Geometry check sheet. Reference: the model listing, model coordinates, mm. Coordinates: 2 decimals unless noted, no trailing zeros. Order: outer loops, then holes, each group sorted by start corner. A loop starts at its lowest first (then second) coordinate and runs counter-clockwise, first axis right, second up. Notation, with made-up numbers: (11, 52) - (17, 52) arc R20 cw to (17, 89) - close; hole circle Ø5 at (61.5, -8). An arc over 180 degrees is marked (long way). Return JSON: item names as keys, results as strings. Group by question number.
Item 1: Draft check along X on faces 1 (the cylindrical face through (0, 11, 1)), 2 (the flat face through (0, 5, 0)), 3 (the cylindrical face through (-0.235, -0.747, 1.479)). Enter one of: pulls with the +X half, pulls with the -X half, needs draft (parallel to the pull), parting line crosses it, or undercut.
Item 2: Gauge pin test, flat end, axial feed: pin 1 (1.5 mm diameter, centred on x = 2, z = 1.5, fed in from +Y). Record the tip position at first contact, or that the pin passes through.
Item 3: Section check A-A on y = 8. Enter the section's corners in (x, z), then the cut area to 3 significant figures.
Item 4: Section check C-C on z = 0.7. Give the number of separate pieces and of enclosed holes in the cut face, then the cut area to 3 significant figures.
Item 5: Scan lines: probe 1 along Y at (x, z) = (0, 0.7); probe 2 along Y at (x, z) = (-0.25, 0.2); probe 3 along X at (y, z) = (7.25, 0.3). Record each from-to range of solid material in increasing order.
Item 6: Section check B-B on x = 0. Enter the section's corners in (y, z).
Item 7: Section check D-D on y = 0.5. Enter the section's corners in (x, z).
Autodesk Inventor part; units mm, degrees
ref_plane "Work Plane2" through (1.7501, 9.2049, 0) normal (0.6132, -0.7899, 0) x (0, 0, 1)
ref_plane "YZ Plane" through (0, 0, 0) normal (1, 0, 0) x (0, 1, 0)
ref_plane "XZ Plane" through (0, 0, 0) normal (0, 1, 0) x (-1, 0, 0)
sketch "Sketch1" plane through (0, 0, 0) normal (0, 0, 1) x (1, 0, 0)
  arc A0 (-1.9843, -0.25) -> (1.9843, -0.25) centre (0, 0) ccw
  arc A1 (2.9765, 7.625) -> (-2.9765, 7.625) centre (0, 8) ccw
  line L0 (2.9765, 7.625) -> (1.9843, -0.25)
  line L1 (-2.9765, 7.625) -> (-1.9843, -0.25)
  circle A2 centre (0, 8) radius 1.5
  dimension "d0" = 3
  dimension "d1" = 2
  dimension "d2" = 8
  dimension "d3" = 3
extrude "Extrusion1" add sketch "Sketch1" along normal blind 3
sketch "Sketch2" plane through (0, 0, 3) normal (0, 0, 1) x (1, 0, 0)
  arc A0 (-1.9843, -0.25) -> (1.9843, -0.25) centre (0, 0) ccw
hole "Hole1" at (0, 0, 3) direction (0, 0, -1) diameter 1.567 end through all
ref_plane "Work Plane2" through (1.7501, 9.2049, 0) normal (0.6132, -0.7899, 0) x (0, 0, 1)
ref_plane "Work Plane1" through (2.9765, 7.625, 0) normal (0.6132, -0.7899, 0) x (0, 0, 1)
sketch "Sketch3" plane through (1.7501, 9.2049, 0) normal (0.6132, -0.7899, 0) x (0, 0, 1)
  line L0 (0, 5.6125) -> (0, 0)
  line L1 (0, 0) -> (0, 4.7025)
  line L2 (0, 4.7025) -> (3, 4.7025)
  line L3 (3, 0) -> (3, 4.7025)
  line L4 (0, 0) -> (3, 0)
  line L5 (0, -0.8787) -> (3, -0.8787)
  point P0 (0, 7.0267)
  point P1 (1.5, 2.1213)
  point P2 (1.5, -0.8787)
  dimension "d15" = 1.5
  dimension "d16" = 3
hole "Hole2" at (0.0744, 7.9042, 1.5) direction (0.6132, -0.7899, 0) diameter 1.1835 end through all
chamfer "Chamfer1" distance 0.1 angle 45 8 edges at (0, 11, 3) (-2.4804, 3.6875, 3) (0, -2, 3) (2.4804, 3.6875, 3) (2.4804, 3.6875, 0) (0, 11, 0) (-2.4804, 3.6875, 0) (0, -2, 0)
properties part number "27 - Valve Level" material "Steel AISI 1020 108 ANLD"
Computed:
{
 "1": {"face 1": "parting line crosses it", "face 2": "needs draft", "face 3": "undercut"},
 "2": {"pin 1": "stops at y = 10.73"},
 "3": {"outline": "(-3, 0.1) - (-2.9, 0) - (-1.5, 0) - (-1.5, 3) - (-2.9, 3) - (-3, 2.9) - close; (1.5, 0) - (2.9, 0) - (3, 0.1) - (3, 2.9) - (2.9, 3) - (1.5, 3) - close", "area": "8.98 mm²"},
 "4": {"separate pieces": "1", "enclosed holes": "2", "area": "51.7 mm²"},
 "5": {"probe 1": "y = -2 to -0.78, 0.78 to 6.5, 9.5 to 11", "probe 2": "y = -1.98 to -0.74, 0.74 to 6.52, 9.48 to 10.99", "probe 3": "x = -2.93 to -1.3, 1.3 to 2.93"},
 "6": {"outline": "(-2, 0.1) - (-1.9, 0) - (-0.78, 0) - (-0.78, 3) - (-1.9, 3) - (-2, 2.9) - close; (0.78, 0) - (6.5, 0) - (6.5, 3) - (0.78, 3) - close; (9.5, 0) - (10.9, 0) - (11, 0.1) - (11, 2.9) - (10.9, 3) - (9.5, 3) - close"},
 "7": {"outline": "(-2.08, 0.1) - (-1.98, 0) - (-0.6, 0) - (-0.6, 3) - (-1.98, 3) - (-2.08, 2.9) - close; (0.6, 0) - (1.98, 0) - (2.08, 0.1) - (2.08, 2.9) - (1.98, 3) - (0.6, 3) - close"}
}
